Verification items for the finished model (mm, model axes). Give positions to 0.01 mm unless a question says otherwise; leave off trailing zeros. Order: outer loops, then holes, each group sorted by start corner. A loop starts at its lowest first (then second) coordinate and runs counter-clockwise, first axis right, second up.
(1) Sectioned sample at B-B on x = 12. Record the cut outline in (y, z), plus the area to 3 significant figures.
(2) Scan lines: L1, parallel to Y at x = 22.5, z = 0.9; L2, parallel to Y at x = -5, z = 0.15. Record each from-to range of solid material in increasing order.
(3) Sectioned sample at A-A on z = 0.4. Record the cut outline in (x, y), plus the area to 3 significant figures.
(4) Sectioned sample at C-C on x = 1.5. Record the cut outline in (y, z).
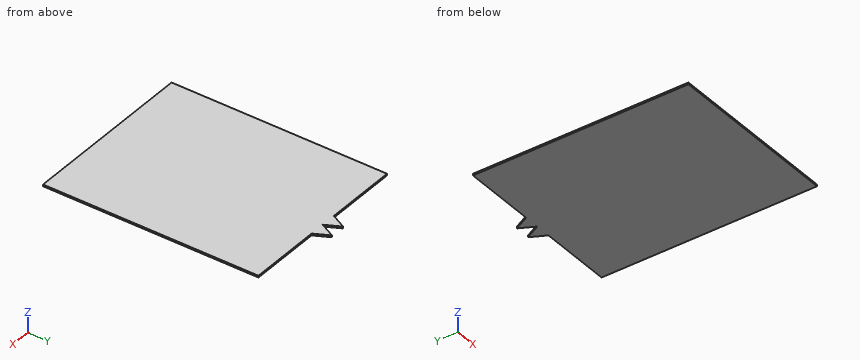
```python
from build123d import *

# Parameters (mm, degrees)
F0_W     = 99
F0_H     = 150
F1_DEPTH = 1
F4_DEPTH = 25


with BuildPart() as f1:
    # F0 (on Top) → F1 (new body)
    with BuildSketch(Plane.XY):
        Rectangle(F0_W, F0_H)
    extrude(amount=F1_DEPTH)

    # F3 (on face) → F4 (cut)
    with BuildSketch(Plane.XY.offset(1)):
        Polygon((-62.001765, 46.220153), (-46.321515, 46.220153), (-8.583423, 46.220153), (-4.291712, 54.622024), (0, 46.220153), (4.291712, 54.622024), (8.583423, 46.220153), (46.321515, 46.220153), (54.136954, 46.220153), (59.024267, 77.810913), (-51.67358, 77.810913), align=None)
    extrude(amount=-F4_DEPTH, mode=Mode.SUBTRACT)


solid = f1.part
```
Ans:
1. outline: (-75, 0) - (46.22, 0) - (46.22, 1) - (-75, 1) - close
1. area: 121 mm2
2. L1: y = -75 to 46.22
2. L2: y = -75 to 53.24
3. outline: (-49.5, -75) - (49.5, -75) - (49.5, 46.22) - (8.58, 46.22) - (4.29, 54.62) - (0, 46.22) - (-4.29, 54.62) - (-8.58, 46.22) - (-49.5, 46.22) - close
3. area: 12,100 mm2
4. outline: (-75, 0) - (49.16, 0) - (49.16, 1) - (-75, 1) - close
